from build123d import *

# Parameters (mm, degrees)
F0_W     = 34.89244
F0_H     = 23.427777
F1_DEPTH = 25.4
F2_R     = 2.80533
F2_R_2   = 2.924594
F3_DEPTH = 34.89344


with BuildPart() as f1:
    # F0 (on Right) → F1 (new body)
    with BuildSketch(Plane.YZ):
        with Locations((17.44622, 11.713888)):
            Rectangle(F0_W, F0_H)
    extrude(amount=F1_DEPTH)

    # F2 (on face) → F3 (cut, through all)
    with BuildSketch(Plane(origin=(0, 34.89244, 0), x_dir=(-1, 0, 0), z_dir=(0, 1, 0))):
        with Locations((-20.318756, 17.947417)):
            Circle(F2_R)
        with Locations((-6.839417, 17.814223)):
            Circle(F2_R_2)
    extrude(amount=-F3_DEPTH, mode=Mode.SUBTRACT)


solid = f1.part
The model under review builds one solid part; all positions refer to its coordinate system, in mm. Give positions to 0.01 mm unless a question says otherwise; leave off trailing zeros. Loops run counter-clockwise (first coordinate to the right, second up) from the corner with the lowest first, then second, coordinate; pieces in that order, holes last. Notation, with made-up numbers: (-3, 61) -> (40, 61) arc R21 ccw to (40, 95) -> close; hole circle Ø7 at (23, 37). An arc over 180 degrees is marked (long way). Put each result on its own line as item: value. Start each with the question number.
1. We need section D-D on x = 21.25. State the section outline as (y, z) points, then the cut area to 3 significant figures.
2. We need section A-A on x = 8. State the section outline as (y, z) points.
3. We need section C-C on y = 26. State the section outline as (x, z) points, then the cut area to 3 significant figures.
4. We need section B-B on z = 16.5. State the section outline as (x, y) points.
5. Wall thickness on probe 1 along X at (y, z) = (2.5, 17.75); probe 2 along X at (y, z) = (17, 20.25); probe 3 along Z at (x, y) = (9, 9.5): over which ranges is each line inside the solid? List them lowest first.
6. Clearance check with flat-ended pins moving along their axes: P1, Ø9, axis at x = 20.32, z = 17.95, coming from the -Y side; P2, Ø3, axis at x = 8, z = 18, coming from the -Y side. State where each tip first meets the part, or that it passes through.
7. Mouldability with a two-part tool opening along X and no side actions: class faces 1 (the face through (17.73, 17.69, 16.87)), 2 (the face through (13, 17, 0)), 3 (the face through (25.4, 17, 12)), 4 (the face through (4.05, 17.69, 18.69)) as released by +X, released by -X, zero draft, split by the parting line, or undercut.
Determined:
1. outline: (0, 0) -> (34.89, 0) -> (34.89, 15.3) -> (0, 15.3) -> close; (0, 20.59) -> (34.89, 20.59) -> (34.89, 23.43) -> (0, 23.43) -> close
1. area: 633 mm^2
2. outline: (0, 0) -> (34.89, 0) -> (34.89, 15.13) -> (0, 15.13) -> close; (0, 20.5) -> (34.89, 20.5) -> (34.89, 23.43) -> (0, 23.43) -> close
3. outline: (0, 0) -> (25.4, 0) -> (25.4, 23.43) -> (0, 23.43) -> close; hole circle Ø5.85 at (6.84, 17.81); hole circle Ø5.61 at (20.32, 17.95)
3. area: 543 mm^2
4. outline: (0, 0) -> (4.23, 0) -> (4.23, 34.89) -> (0, 34.89) -> close; (9.45, 0) -> (17.92, 0) -> (17.92, 34.89) -> (9.45, 34.89) -> close; (22.72, 0) -> (25.4, 0) -> (25.4, 34.89) -> (22.72, 34.89) -> close
5. probe 1: 0 to 3.92, 9.76 to 17.52, 23.12 to 25.4
5. probe 2: 0 to 5.22, 8.46 to 18.72, 21.92 to 25.4
5. probe 3: 0 to 15.84, 19.79 to 23.43
6. P1: y = 0
6. P2: through
7. face 1: undercut
7. face 2: zero draft
7. face 3: released by +X
7. face 4: undercut
